from build123d import *

# Parameters (mm, degrees)
F2_W      = 50
F2_H      = 30
F3_DEPTH  = 30
F0_R      = 8.5
F4_DEPTH  = 20
F5_W      = 5
F5_H      = 30
F6_DEPTH  = 22
F7_W      = 30
F7_H      = 2
F8_DEPTH  = 6
F9_W      = 30
F9_H      = 2
F10_DEPTH = 11
F11_W     = 20
F11_H     = 20
F12_DEPTH = 12.5
F13_W     = 50
F13_H     = 30
F14_DEPTH = 10
F15_DEPTH = 25
F16_R     = 5.25
F17_DEPTH = 50


with BuildPart() as f3:
    # F2 (on offset) → F3 (new body)
    with BuildSketch(Plane.XY.offset(20)):
        Rectangle(F2_W, F2_H)
    extrude(amount=-F3_DEPTH)

    # F0 (on Top) → F4 (cut)
    with BuildSketch(Plane.XY):
        Circle(F0_R)
    extrude(amount=F4_DEPTH, mode=Mode.SUBTRACT)

    # F5 (on face) → F6 (join)
    with BuildSketch(Plane.XY.offset(20)):
        with Locations((-22.5, 0)):
            Rectangle(F5_W, F5_H)
        with Locations((22.5, 0)):
            Rectangle(F5_W, F5_H)
    extrude(amount=F6_DEPTH)

    # F7 (on face) → F8 (join)
    with BuildSketch(Plane.YZ.offset(-20)):
        with Locations((0, 41)):
            Rectangle(F7_W, F7_H)
    extrude(amount=F8_DEPTH)

    # F9 (on face) → F10 (join)
    with BuildSketch(Plane(origin=(20, 0, 0), x_dir=(0, -1, 0), z_dir=(-1, 0, 0))):
        with Locations((0, 41)):
            Rectangle(F9_W, F9_H)
    extrude(amount=F10_DEPTH)

    # F11 (on Top) → F12 (cut, symmetric)
    with BuildSketch(Plane.XY):
        Rectangle(F11_W, F11_H)
    extrude(amount=F12_DEPTH, both=True, mode=Mode.SUBTRACT)

    # F13 (on face) → F14 (join)
    with BuildSketch(Plane(origin=(0, 0, -10), x_dir=(1, 0, 0), z_dir=(0, 0, -1))):
        Rectangle(F13_W, F13_H)
    extrude(amount=F14_DEPTH)

    # F0 (on Top) → F15 (cut)
    with BuildSketch(Plane.XY):
        Circle(F0_R)
    extrude(amount=-F15_DEPTH, mode=Mode.SUBTRACT)

    # F16 (on face) → F17 (cut)
    with BuildSketch(Plane.YZ.offset(25)):
        Circle(F16_R)
    extrude(amount=-F17_DEPTH, mode=Mode.SUBTRACT)


solid = f3.part
For this review, take the finished solid that the model builds, in its own axes (mm). A direction names the side the tool comes from. Coordinates: 2 decimals unless noted, no trailing zeros. Loops run counter-clockwise (first coordinate to the right, second up) from the corner with the lowest first, then second, coordinate; pieces in that order, holes last. Notation, with made-up numbers: (74, -34.5) - (130, -34.5) arc R17 cw to (130, -24.5) - close; hole circle Ø8 at (4, -12.75). An arc over 180 degrees is marked (long way). Use a Markdown table: item, result. Add a question column.
Item 1: We need section A-A (z = 0). Give the boundary of the cut face in (x, y).
Item 2: Insertion check: pin 1 Ø9.5 at (y, z) = (0, 0) entering from +X. The pin has a flat end and moves straight along its axis. Give the tip position at first contact, or say it passes through.
Item 3: Tool access review of faces 1 (the face through (9, 0, 20)), 2 (the face through (0, -15, 5)), 3 (the face through (-10, 0, 6)), 4 (the face through (-14, 0, 41)): name each direction out of +Z, -Z, +X, -X, +Y, -Y from which nothing blocks a thin tool from reaching the whole face with its end or side.
Item 4: We need section D-D (z = -14.5). Give the boundary of the cut face in (x, y), and give its area (3 significant figures).
Item 5: We need section C-C (x = 0). Give the boundary of the cut face in (y, z), and give its area (4 significant figures).
Item 6: We need section B-B (y = 0). Give the number of separate pieces and of enclosed holes in the cut face, and give its area (3 significant figures).
Item 7: For line 1 (Z direction, x = 18.5, y = 0); line 2 (X direction, y = 0, z = 14.5); line 3 (Z direction, x = 17.5, y = 6), list the stretches that pass through material, from the lowest coordinate up.
Item 8: Mouldability with a two-part tool opening along X and no side actions: class faces 5 (the face through (20, 0, 30)), 6 (the face through (17, 0, 42)), 7 (the face through (-25, 0, 11)), 8 (the face through (25, 0, 11)) as pulls with the +X half, pulls with the -X half, needs draft (parallel to the pull), parting line crosses it, or undercut.
Results list:
| question | item | result |
|---|---|---|
| 1 | outline | (-25, -15) - (25, -15) - (25, -5.25) - (10, -5.25) - (10, -10) - (-10, -10) - (-10, -5.25) - (-25, -5.25) - close; (-25, 5.25) - (-10, 5.25) - (-10, 10) - (10, 10) - (10, 5.25) - (25, 5.25) - (25, 15) - (-25, 15) - close |
| 2 | pin 1 | passes through |
| 3 | face 1 | +Y, -Y |
| 3 | face 2 | +Z, -Z, +X, -X, -Y |
| 3 | face 3 | none |
| 3 | face 4 | +Z, +Y, -Y |
| 4 | outline | (-25, -15) - (25, -15) - (25, 15) - (-25, 15) - close; hole circle Ø17 at (0, 0) |
| 4 | area | 1,270 mm^2 |
| 5 | outline | (-15, -20) - (-8.5, -20) - (-8.5, -10) - (-10, -10) - (-10, 12.5) - (-8.5, 12.5) - (-8.5, 20) - (-15, 20) - close; (8.5, -20) - (15, -20) - (15, 20) - (8.5, 20) - (8.5, 12.5) - (10, 12.5) - (10, -10) - (8.5, -10) - close |
| 5 | area | 452.5 mm^2 |
| 6 | separate pieces | 4 |
| 6 | enclosed holes | 0 |
| 6 | area | 1,190 mm^2 |
| 7 | line 1 | z = -20 to -5.25, 5.25 to 20, 40 to 42 |
| 7 | line 2 | x = -25 to -8.5, 8.5 to 25 |
| 7 | line 3 | z = -20 to 20, 40 to 42 |
| 8 | face 5 | undercut |
| 8 | face 6 | needs draft |
| 8 | face 7 | pulls with the -X half |
| 8 | face 8 | pulls with the +X half |
